from build123d import *

# Parameters (mm, degrees)
CROQUIS1_R              = 1.5
SALIENTE_EXTRUIR1_DEPTH = 1.5


with BuildPart() as part:
    # Croquis1 → Saliente-Extruir1 (new, symmetric)
    # profile 1 of 4: a face of its own
    with BuildSketch(Plane.XY):
        with BuildLine():
            Line((-4, 24.5), (-4, -17.5))
            Line((-4, -17.5), (4, -17.5))
            Line((4, -17.5), (4, 24.5))
            ThreePointArc((4, 24.5), (3.121320344, 26.621320344), (1, 27.5))
            Line((1, 27.5), (-1, 27.5))
            ThreePointArc((-1, 27.5), (-3.121320344, 26.621320344), (-4, 24.5))
        make_face()
        with Locations((0, 22.5)):
            Circle(CROQUIS1_R, mode=Mode.SUBTRACT)
    # profile 2 of 4: a face of its own
    with BuildSketch(Plane.XY):
        with BuildLine():
            Line((-6, -27.5), (-1, -27.5))
            ThreePointArc((-1, -27.5), (-3.121320344, -26.621320344), (-4, -24.5))
            Line((-4, -24.5), (-4, -17.5))
            Line((-4, -17.5), (-6, -17.5))
            ThreePointArc((-6, -17.5), (-8.121320344, -18.378679656), (-9, -20.5))
            Line((-9, -20.5), (-9, -24.5))
            ThreePointArc((-9, -24.5), (-8.121320344, -26.621320344), (-6, -27.5))
        make_face()
        with Locations((-6, -22.5)):
            Circle(CROQUIS1_R, mode=Mode.SUBTRACT)
    # profile 3 of 4: a face of its own
    with BuildSketch(Plane.XY):
        with BuildLine():
            ThreePointArc((-4, -24.5), (-3.121320344, -26.621320344), (-1, -27.5))
            Line((-1, -27.5), (1, -27.5))
            ThreePointArc((1, -27.5), (3.121320344, -26.621320344), (4, -24.5))
            Line((4, -24.5), (4, -17.5))
            Line((4, -17.5), (-4, -17.5))
            Line((-4, -17.5), (-4, -24.5))
        make_face()
    # profile 4 of 4: a face of its own
    with BuildSketch(Plane.XY):
        with BuildLine():
            ThreePointArc((4, -24.5), (3.121320344, -26.621320344), (1, -27.5))
            Line((1, -27.5), (6, -27.5))
            ThreePointArc((6, -27.5), (8.121320344, -26.621320344), (9, -24.5))
            Line((9, -24.5), (9, -20.5))
            ThreePointArc((9, -20.5), (8.121320344, -18.378679656), (6, -17.5))
            Line((6, -17.5), (4, -17.5))
            Line((4, -17.5), (4, -24.5))
        make_face()
        with Locations((6, -22.5)):
            Circle(CROQUIS1_R, mode=Mode.SUBTRACT)
    extrude(amount=SALIENTE_EXTRUIR1_DEPTH, both=True)


solid = part.part
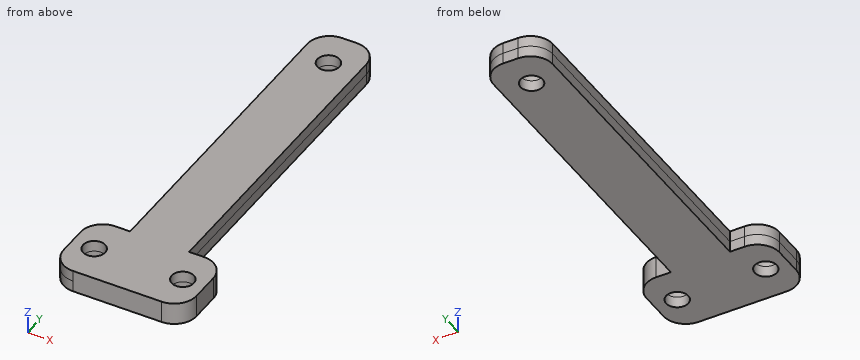
Work out the finished part from the listing and answer in its coordinate system (mm). Give positions to 0.01 mm unless a question says otherwise; leave off trailing zeros. Loops run counter-clockwise (first coordinate to the right, second up) from the corner with the lowest first, then second, coordinate; pieces in that order, holes last. Notation, with made-up numbers: (-37, 39.25) - (7, 39.25) arc R10 cw to (7, 58.25) - close; hole circle Ø7 at (1.25, -3.75). An arc over 180 degrees is marked (long way). Answer in a Markdown table with one row per item.
(1) Section D-D (y = 22.5) is taken. Give the vertices of the cut face in (x, z), and give its area (3 significant figures).
Results list:
| item | result |
|---|---|
| outline | (-4, -1.5) - (-1.5, -1.5) - (-1.5, 1.5) - (-4, 1.5) - close; (1.5, -1.5) - (4, -1.5) - (4, 1.5) - (1.5, 1.5) - close |
| area | 15.0 mm² |
(2) Section B-B (z = -0.85) is taken. Give the vertices of the cut face in (x, y).
Results list:
| item | result |
|---|---|
| outline | (-9, -24.5) arc R3 ccw to (-6, -27.5) - (6, -27.5) arc R3 ccw to (9, -24.5) - (9, -20.5) arc R3 ccw to (6, -17.5) - (4, -17.5) - (4, 24.5) arc R3 ccw to (1, 27.5) - (-1, 27.5) arc R3 ccw to (-4, 24.5) - (-4, -17.5) - (-6, -17.5) arc R3 ccw to (-9, -20.5) - close; hole circle Ø3 at (-6, -22.5); hole circle Ø3 at (0, 22.5); hole circle Ø3 at (6, -22.5) |
(3) Flat-ended cylindrical pins translate along their axes: pin 1 Ø0.8 at (x, z) = (-5.5, 1) entering from +Y; pin 2 Ø1.8 at (x, y) = (-6, -22.5) entering from -Z; pin 3 Ø4 at (x, y) = (0, 22.5) entering from -Z; pin 4 Ø1.2 at (y, z) = (-3, -0.5) entering from -X. Find the tip coordinate at first contact, or state that the pin passes through.
Results list:
| item | result |
|---|---|
| pin 1 | stops at y = -17.5 |
| pin 2 | passes through |
| pin 3 | stops at z = -1.5 |
| pin 4 | stops at x = -4 |
(4) Consider L1, parallel to Y at x = 6, z = -1.2; L2, parallel to Y at x = -6.5, z = -0.8; L3, parallel to X at y = -8, z = -0.1. Determine where each line is inside the solid, lowest interval first. Write a range as [from, to].
Results list:
| item | result |
|---|---|
| L1 | y = [-27.5, -24], [-21, -17.5] |
| L2 | y = [-27.46, -23.91], [-21.09, -17.54] |
| L3 | x = [-4, 4] |
(5) Section A-A (x = 0) is taken. Give the vertices of the cut face in (y, z), and give its area (3 significant figures).
Results list:
| item | result |
|---|---|
| outline | (-27.5, -1.5) - (21, -1.5) - (21, 1.5) - (-27.5, 1.5) - close; (24, -1.5) - (27.5, -1.5) - (27.5, 1.5) - (24, 1.5) - close |
| area | 156 mm² |
(6) Section C-C (y = -22.5) is taken. Give the vertices of the cut face in (x, z).
Results list:
| item | result |
|---|---|
| outline | (-9, -1.5) - (-7.5, -1.5) - (-7.5, 1.5) - (-9, 1.5) - close; (-4.5, -1.5) - (4.5, -1.5) - (4.5, 1.5) - (-4.5, 1.5) - close; (7.5, -1.5) - (9, -1.5) - (9, 1.5) - (7.5, 1.5) - close |
